Geometry: final body of the model. Coordinates: model frame, mm. Coordinates: 2 decimals unless noted, no trailing zeros. Order: outer loops, then holes, each group sorted by start corner. A loop starts at its lowest first (then second) coordinate and runs counter-clockwise, first axis right, second up. Notation, with made-up numbers: M 58,-37.75 L 73,-37.75 A16 ccw 73,-27.75 Z; hole C -38.5,-13 d3. An arc over 180 degrees is marked long. Use CSV: the item, a comma, the result in double quotes. Start each with the question number.
1. Material intervals for line 1 (Y direction, x = 0, z = 0.95); line 2 (X direction, y = -8.5, z = 1.75); line 3 (X direction, y = 10.5, z = 0.35), sorted ascending.
2. Section query A-A on y = 0. Return the cut outline in (x, z).
3. First-contact query: P1, Ø1.5, axis at x = -1, y = 10, coming from the -Z side; P2, Ø8, axis at x = 4.5, y = 7.5, coming from the -Z side. Flat tips, straight axial feed; report the tip coordinate or a pass-through.
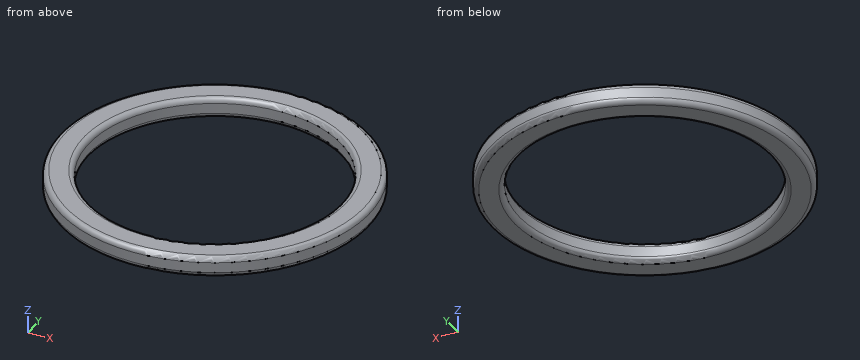
from build123d import *

# Parameters (mm, degrees)
SKETCH1_R           = 15
SKETCH1_R_2         = 12.25
BOSS_EXTRUDE1_DEPTH = 2
FILLET1_R           = 0.5
FILLET2_R           = 0.5
FILLET3_R           = 0.5


with BuildPart() as part:
    # Sketch1 → Boss-Extrude1 (new body)
    with BuildSketch(Plane.XY):
        Circle(SKETCH1_R)
        Circle(SKETCH1_R_2, mode=Mode.SUBTRACT)
    extrude(amount=BOSS_EXTRUDE1_DEPTH)

    # Fillet1
    fillet1_edges = [part.edges().sort_by_distance(p)[0] for p in [
        (-15, 0, 2),
        (-12.25, 0, 2),
    ]]
    fillet(fillet1_edges, radius=FILLET1_R)

    # Fillet2
    fillet2_edges = [part.edges().sort_by_distance(p)[0] for p in [
        (-15, 0, 0),
    ]]
    fillet(fillet2_edges, radius=FILLET2_R)

    # Fillet3
    fillet3_edges = [part.edges().sort_by_distance(p)[0] for p in [
        (-12.25, 0, 0),
    ]]
    fillet(fillet3_edges, radius=FILLET3_R)


solid = part.part
Results list:
1,line 1,"y = -15 to -12.25, 12.25 to 15"
1,line 2,"x = -12.28 to -8.91, 8.91 to 12.28"
1,line 3,"x = -10.68 to -6.35, 6.35 to 10.68"
2,outline,"M -15,0.5 A0.5 ccw -14.5,0 L -12.75,0 A0.5 ccw -12.25,0.5 L -12.25,1.5 A0.5 ccw -12.75,2 L -14.5,2 A0.5 ccw -15,1.5 Z; M 12.25,0.5 A0.5 ccw 12.75,0 L 14.5,0 A0.5 ccw 15,0.5 L 15,1.5 A0.5 ccw 14.5,2 L 12.75,2 A0.5 ccw 12.25,1.5 Z"
3,P1,"passes through"
3,P2,"stops at z = 0"
